Geometry: final body of the model. Coordinates: model frame, mm. A direction names the side the tool comes from. Give positions to 0.01 mm unless a question says otherwise; leave off trailing zeros. Write each loop counter-clockwise with the first axis right and the second up, starting at its lowest first coordinate (ties: lowest second). Pieces come first, ordered by that corner, then holes. Notation, with made-up numbers: M 33,-11.75 L 71,-11.75 A10 ccw 71,2.25 Z; hole C 45,14 d10. An arc over 180 degrees is marked long. Use a Markdown table: item, result. Add a question column.
(1) Material intervals for L1, parallel to X at y = -33, z = 13 (3 decimals); L2, parallel to X at y = -42, z = -16 (3 decimals); L3, parallel to Z at x = 17.5, y = -27, sorted ascending.
(2) Draft query along Z for faces 1 (the flat face through (0, -42, -25.4)), 2 (the flat face through (28.575, -42, 0)), 3 (the flat face through (-15, -43, 23.348)). Return one class per face: released by +Z, released by -Z, zero draft, split by the parting line, or undercut.
(3) Pin query (flat end, axial travel): pin 1 Ø12 at (x, z) = (21.5, -7) entering from +Y; pin 2 Ø4 at (x, z) = (5.5, -18.5) entering from -Y. Return the tip coordinate at first contact, or that it passes through.
(4) Reachability of faces 4 (the flat face through (14, -43, -0.483)), 5 (the flat face through (0, 0, 4)) from +Z, -Z, +X, -X, +Y, -Y: full face, straight path, thin tool, end or side. Return the list, or none.
(5) Cut plane B-B (z = 7). Output: boundary loops of the cut face in (x, y) (3 decimals).
(6) Cut plane C-C (y = -29). Output: boundary loops of the cut face in (x, z) (3 decimals), plus the area to 3 significant figures.
(7) Cut plane A-A (x = -7). Output: boundary loops of the cut face in (y, z) (3 decimals).
```python
from build123d import *

# Parameters (mm, degrees)
F0_W     = 57.15
F0_H     = 50.8
F1_DEPTH = 85.725
F2_W     = 23.8125
F2_H     = 23.8252
F3_DEPTH = 85.726
F4_W     = 23.8125
F4_H     = 23.8252
F5_DEPTH = 85.726
F6_W     = 23.8125
F6_H     = 23.8252
F7_DEPTH = 85.726
F8_W     = 23.8125
F8_H     = 23.8252
F9_DEPTH = 85.726


with BuildPart() as f1:
    # F0 (on Front) → F1 (new body)
    with BuildSketch(Plane.XZ):
        Rectangle(F0_W, F0_H)
    extrude(amount=F1_DEPTH)

    # F2 (on face) → F3 (cut, through all)
    with BuildSketch(Plane.XZ.offset(85.725)):
        with Locations((-14.643011, 11.435687)):
            Rectangle(F2_W, F2_H)
    extrude(amount=-F3_DEPTH, mode=Mode.SUBTRACT)

    # F4 (on face) → F5 (cut, through all)
    with BuildSketch(Plane.XZ.offset(85.725)):
        with Locations((14.437895, 11.43)):
            Rectangle(F4_W, F4_H)
    extrude(amount=-F5_DEPTH, mode=Mode.SUBTRACT)

    # F6 (on face) → F7 (cut, through all)
    with BuildSketch(Plane.XZ.offset(85.725)):
        with Locations((-14.638421, -12.833685)):
            Rectangle(F6_W, F6_H)
    extrude(amount=-F7_DEPTH, mode=Mode.SUBTRACT)

    # F8 (on face) → F9 (cut, through all)
    with BuildSketch(Plane.XZ.offset(85.725)):
        with Locations((14.337632, -12.833685)):
            Rectangle(F8_W, F8_H)
    extrude(amount=-F9_DEPTH, mode=Mode.SUBTRACT)


solid = f1.part
```
Answer list:
| question | item | result |
|---|---|---|
| 1 | L1 | -28.575 to -26.549, -2.737 to 2.532, 26.344 to 28.575 |
| 1 | L2 | -28.575 to -26.545, -2.732 to 2.431, 26.244 to 28.575 |
| 1 | L3 | -25.4 to -24.75, -0.92 to -0.48, 23.34 to 25.4 |
| 2 | face 1 | released by -Z |
| 2 | face 2 | zero draft |
| 2 | face 3 | undercut |
| 3 | pin 1 | y = 0 |
| 3 | pin 2 | through |
| 4 | face 4 | +Y, -Y |
| 4 | face 5 | +Z, -Z, +X, -X, +Y |
| 5 | outline | M -28.575,-85.725 L -26.549,-85.725 L -26.549,0 L -28.575,0 Z; M -2.737,-85.725 L 2.532,-85.725 L 2.532,0 L -2.737,0 Z; M 26.344,-85.725 L 28.575,-85.725 L 28.575,0 L 26.344,0 Z |
| 6 | outline | M -28.575,-25.4 L 28.575,-25.4 L 28.575,25.4 L -28.575,25.4 Z; hole M -26.549,-0.477 L -2.737,-0.477 L -2.737,23.348 L -26.549,23.348 Z; hole M -26.545,-24.746 L -2.732,-24.746 L -2.732,-0.921 L -26.545,-0.921 Z; hole M 2.431,-24.746 L 26.244,-24.746 L 26.244,-0.921 L 2.431,-0.921 Z; hole M 2.532,-0.483 L 26.344,-0.483 L 26.344,23.343 L 2.532,23.343 Z |
| 6 | area | 634 mm² |
| 7 | outline | M -85.725,-25.4 L 0,-25.4 L 0,-24.746 L -85.725,-24.746 Z; M -85.725,-0.921 L 0,-0.921 L 0,-0.477 L -85.725,-0.477 Z; M -85.725,23.348 L 0,23.348 L 0,25.4 L -85.725,25.4 Z |
